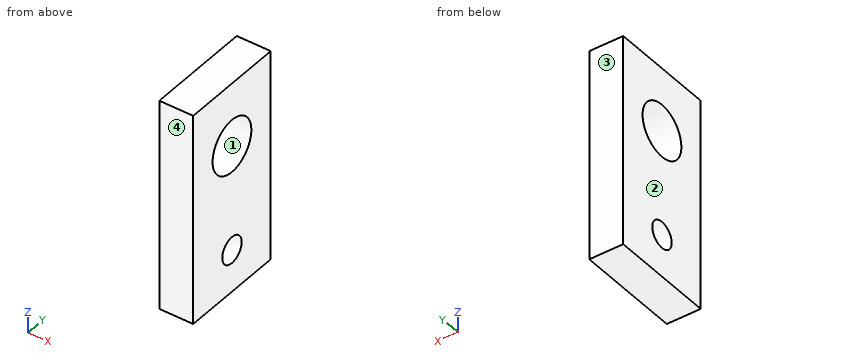
from build123d import *

# Parameters (mm, degrees)
SKETCH1_W                          = 12.7
SKETCH1_H                          = 6.35
BOSS_EXTRUDE1_DEPTH                = 2.032
F_1_16_0_0625_DIAMETER_HOLE1_D     = 1.5875
F_1_16_0_0625_DIAMETER_HOLE1_DEPTH = 70.104
F_1_16_0_0625_DIAMETER_HOLE1_TIP   = 0.476933116
F_1_8_0_125_DIAMETER_HOLE1_D       = 3.175
F_1_8_0_125_DIAMETER_HOLE1_DEPTH   = 70.104
F_1_8_0_125_DIAMETER_HOLE1_TIP     = 0.953866233


with BuildPart() as part:
    # Sketch1 → Boss-Extrude1 (new body)
    with BuildSketch(Plane(origin=(0, 0, 0), x_dir=(0, 0, -1), z_dir=(1, 0, 0))):
        with Locations((6.35, 3.175)):
            Rectangle(SKETCH1_W, SKETCH1_H)
    extrude(amount=BOSS_EXTRUDE1_DEPTH)

    # 1/16 (0.0625) Diameter Hole1
    with Locations(Plane(origin=(2.032, 0, 0), x_dir=(0, 0, -1), z_dir=(1, 0, 0))):
        with Locations((10.16, 3.175)):
            Hole(F_1_16_0_0625_DIAMETER_HOLE1_D / 2, depth=F_1_16_0_0625_DIAMETER_HOLE1_DEPTH)
            with Locations((0, 0, -(F_1_16_0_0625_DIAMETER_HOLE1_DEPTH + F_1_16_0_0625_DIAMETER_HOLE1_TIP / 2))):  # 118° drill point
                Cone(0, F_1_16_0_0625_DIAMETER_HOLE1_D / 2, F_1_16_0_0625_DIAMETER_HOLE1_TIP, mode=Mode.SUBTRACT)

    # 1/8 (0.125) Diameter Hole1
    with Locations(Plane(origin=(2.032, 0, 0), x_dir=(0, 0, -1), z_dir=(1, 0, 0))):
        with Locations((3.81, 3.175)):
            Hole(F_1_8_0_125_DIAMETER_HOLE1_D / 2, depth=F_1_8_0_125_DIAMETER_HOLE1_DEPTH)
            with Locations((0, 0, -(F_1_8_0_125_DIAMETER_HOLE1_DEPTH + F_1_8_0_125_DIAMETER_HOLE1_TIP / 2))):  # 118° drill point
                Cone(0, F_1_8_0_125_DIAMETER_HOLE1_D / 2, F_1_8_0_125_DIAMETER_HOLE1_TIP, mode=Mode.SUBTRACT)


solid = part.part
Geometry: final body of the model. Coordinates: model frame, mm. Face numbers are marked on the shaded views. Give positions to 0.01 mm unless a question says otherwise; leave off trailing zeros. Write each loop counter-clockwise with the first axis right and the second up, starting at its lowest first coordinate (ties: lowest second). Pieces come first, ordered by that corner, then holes. Notation, with made-up numbers: (-18, -28) - (16, -28) arc R22 ccw to (16, 8) - close; hole circle Ø7 at (2, 26). An arc over 180 degrees is marked (long way). Return JSON: item names as keys, results as strings. Group by question number.
1) Section D-D on x = 1.45. State how many separate pieces and enclosed holes the cut face has, plus the area to 3 significant figures.
2) Section C-C on y = 4.5. Return the cut outline in (x, z).
3) Section A-A on z = -3.81. Return the cut outline in (x, y).
4) Section B-B on y = 3. Return the cut outline in (x, z), plus the area to 3 significant figures.
5) Mould query, pull axis Y, two halves, no side actions, for the marked faces 1, 2, 3 and 4. Classes: released by +Y, released by -Y, zero draft, split by the parting line, or undercut.
6) Line query: line 1 (Y direction, x = 1.4, z = -10.16); line 2 (Y direction, x = 0.85, z = -3.81); line 3 (Z direction, x = 0.75, y = 2.75). Output: solid intervals per line, ascending.
Filled in:
{
 "1": {"separate pieces": "1", "enclosed holes": "2", "area": "70.7 mm^2"},
 "2": {"outline": "(0, -12.7) - (2.03, -12.7) - (2.03, -4.68) - (0, -4.68) - close; (0, -2.94) - (2.03, -2.94) - (2.03, 0) - (0, 0) - close"},
 "3": {"outline": "(0, 0) - (2.03, 0) - (2.03, 1.59) - (0, 1.59) - close; (0, 4.76) - (2.03, 4.76) - (2.03, 6.35) - (0, 6.35) - close"},
 "4": {"outline": "(0, -12.7) - (2.03, -12.7) - (2.03, -10.93) - (0, -10.93) - close; (0, -9.39) - (2.03, -9.39) - (2.03, -5.39) - (0, -5.39) - close; (0, -2.23) - (2.03, -2.23) - (2.03, 0) - (0, 0) - close", "area": "16.2 mm^2"},
 "5": {"face 1": "undercut", "face 2": "zero draft", "face 3": "released by +Y", "face 4": "released by -Y"},
 "6": {"line 1": "y = 0 to 2.38, 3.97 to 6.35", "line 2": "y = 0 to 1.59, 4.76 to 6.35", "line 3": "z = -12.7 to -10.83, -9.49 to -5.34, -2.28 to 0"}
}
